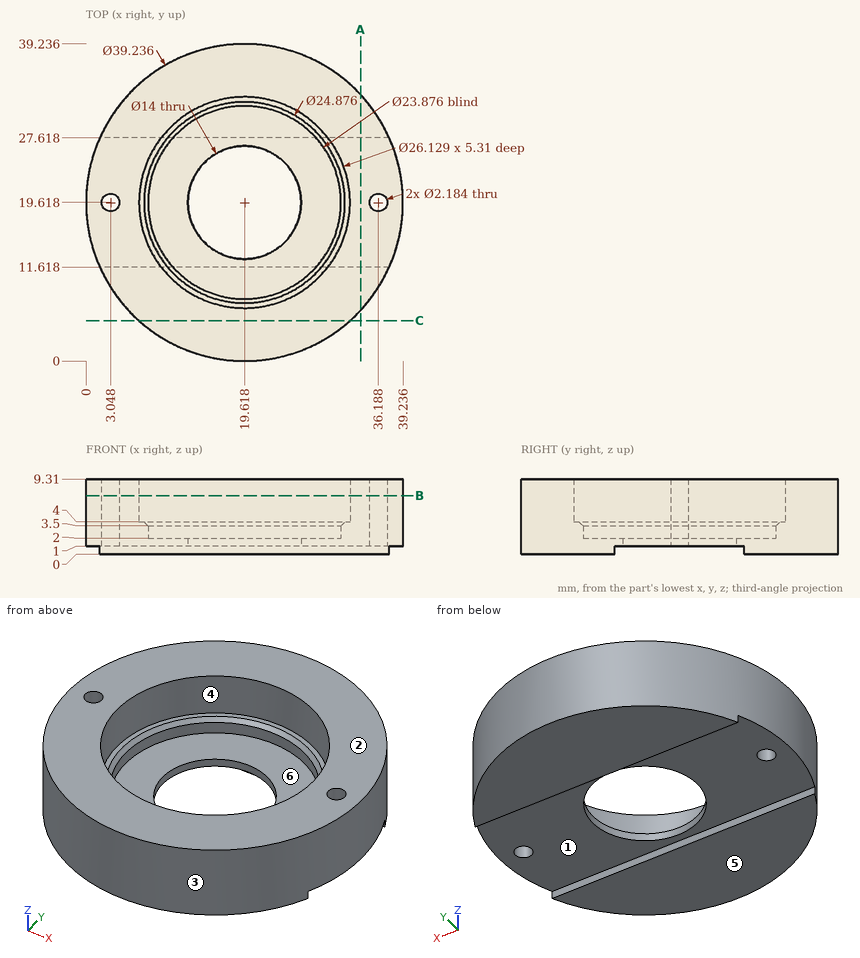
For this review, use the dimensioned drawing (mm, ordinates from the lowest corner) and the shaded views. A direction names the side the tool comes from. Give positions to 0.01 mm unless a question says otherwise; leave off trailing zeros. Order: outer loops, then holes, each group sorted by start corner. A loop starts at its lowest first (then second) coordinate and runs counter-clockwise, first axis right, second up. Notation, with made-up numbers: (70.25, 66.25) -> (106.25, 66.25) arc R20 cw to (106.25, 82.25) -> close; hole circle Ø5 at (70.25, 6). An arc over 180 degrees is marked (long way). Write item = value, one per line. Start each with the question number.
(1) Take a section at C-C (y = 5). Write out the cut boundary in (x, z) (1 decimal), plus the area to 3 significant figures.
(2) Tool access review of the marked faces 1 and 2: name each direction out of +Z, -Z, +X, -X, +Y, -Y from which nothing blocks a thin tool from reaching the whole face with its end or side.
(3) For L1, parallel to Z at x = 2.5, y = 22; L2, parallel to Y at x = 20, z = 3.25; L3, parallel to X at y = 17, z = 8 (1 decimal), list the stretches that pass through material, from the lowest coordinate up. Write a range as from..to.
(4) Draft analysis for pull direction X (two halves, no side actions). For the marked faces 3, 4, 5 and 6, state which applies: +X half, -X half, draft (parallel to the pull), parting line (faces both ways), or undercut.
(5) For pin 1 Ø7 at (x, y) = (20, 16) entering from +Z; pin 2 Ø3 at (y, z) = (23.5, 7.5) entering from +X; pin 3 Ø2 at (x, z) = (17.5, 8.5) entering from +Y; pin 4 Ø8 at (x, y) = (10.5, 27.5) entering from +Z, all flat-tipped, find the tip position at first contact; note any pin that passes through.
(6) Take a section at B-B (z = 7.25). Write out the cut boundary in (x, y) (1 decimal).
(7) Take a section at A-A (x = 34). Write out the cut boundary in (y, z) (1 decimal).
Returned:
q1.outline = (6.5, 0) -> (32.7, 0) -> (32.7, 9.3) -> (6.5, 9.3) -> close
q1.area = 244 mm²
q2.face_1 = -Z, +X, -X
q2.face_2 = +Z, +X, -X, +Y, -Y
q3.L1 = 1..9.31
q3.L2 = 0..7.69, 31.55..39.23
q3.L3 = 0.2..6.8, 32.4..39.1
q4.face_3 = parting line
q4.face_4 = undercut
q4.face_5 = draft
q4.face_6 = undercut
q5.pin_1 = 2
q5.pin_2 = 39.09
q5.pin_3 = 39.2
q5.pin_4 = 9.31
q6.outline = circle Ø39.2 at (19.6, 19.6); hole circle Ø2.2 at (3, 19.6); hole circle Ø26.1 at (19.6, 19.6); hole circle Ø2.2 at (36.2, 19.6)
q7.outline = (6.3, 0) -> (11.6, 0) -> (11.6, 1) -> (27.6, 1) -> (27.6, 0) -> (33, 0) -> (33, 9.3) -> (6.3, 9.3) -> close
